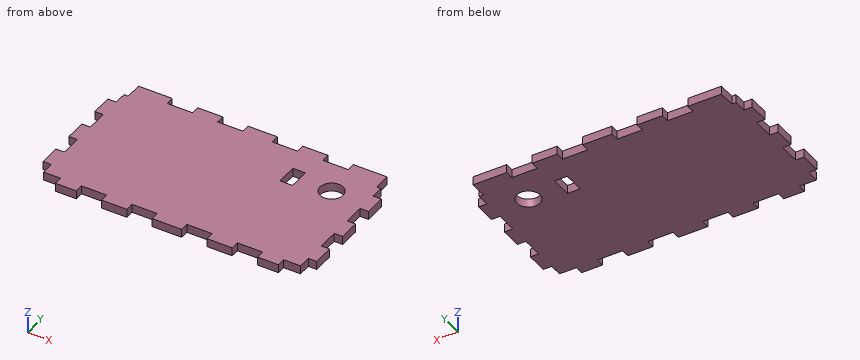
Autodesk Inventor part; units mm, degrees
ref_plane "YZ Plane" through (0, 0, 0) normal (1, 0, 0) x (0, 1, 0)
ref_plane "XZ Plane" through (0, 0, 0) normal (0, 1, 0) x (-1, 0, 0)
ref_plane "XY Plane" through (0, 0, 0) normal (0, 0, 1) x (1, 0, 0)
sketch "Sketch1" plane through (0, 0, 0) normal (0, 0, 1) x (1, 0, 0)
  line L0 (0, -74) -> (130, -74)
  line L1 (130, -74) -> (130, 0)
  line L2 (130, 0) -> (0, 0)
  line L3 (0, 0) -> (0, -74)
  dimension "d228" = 130
  dimension "d229" = 74
extrude "Extrusion1" add sketch "Sketch1" against normal blind 4
sketch "Sketch2" plane through (0, 0, 0) normal (0, 0, 1) x (1, 0, 0)
  line L0 (0, -74) -> (0, 0)
  line L1 (0, -37) -> (130, -37)
  line L2 (130, 0) -> (130, -74)
  line L3 (65, 0) -> (65, -74)
  line L4 (130, -74) -> (0, -74)
  line L5 (22, -74) -> (12, -74)
  line L6 (12, -74) -> (12, -70)
  line L7 (22, -70) -> (22, -74)
  line L8 (46, -70) -> (46, -74)
  line L9 (46, -74) -> (34, -74)
  line L10 (34, -74) -> (34, -70)
  line L11 (72, -70) -> (72, -74)
  line L12 (72, -74) -> (58, -74)
  line L13 (58, -74) -> (58, -70)
  line L14 (0, -74) -> (130, -74)
  line L15 (96, -74) -> (84, -74)
  line L16 (84, -74) -> (84, -70)
  line L17 (96, -70) -> (96, -74)
  line L18 (118, -70) -> (118, -74)
  line L19 (118, -74) -> (108, -74)
  line L20 (108, -74) -> (108, -70)
  line L21 (0, -54) -> (4, -54)
  line L22 (4, -54) -> (4, -44)
  line L23 (4, -44) -> (0, -44)
  line L24 (0, -44) -> (0, -54)
  line L25 (0, -34) -> (4, -34)
  line L26 (4, -34) -> (4, -24)
  line L27 (4, -24) -> (0, -24)
  line L28 (0, -24) -> (0, -34)
  line L29 (0, 0) -> (0, -74)
  line L30 (130, -74) -> (130, 0)
  line L31 (130, 0) -> (130, -74)
  line L32 (0, -70) -> (12, -70)
  line L33 (22, -70) -> (34, -70)
  line L34 (46, -70) -> (58, -70)
  line L35 (72, -70) -> (84, -70)
  line L36 (96, -70) -> (108, -70)
  line L37 (118, -70) -> (130, -70)
  line L38 (0, 0) -> (0, -74)
  line L39 (6, 0) -> (6, -8)
  line L40 (22, -4) -> (22, 0)
  line L41 (46, -4) -> (46, 0)
  line L42 (46, 0) -> (34, 0)
  line L43 (34, 0) -> (34, -4)
  line L44 (72, -4) -> (72, 0)
  line L45 (72, 0) -> (58, 0)
  line L46 (58, 0) -> (58, -4)
  line L47 (96, -4) -> (96, 0)
  line L48 (108, 0) -> (108, -4)
  line L49 (96, 0) -> (84, 0)
  line L50 (84, 0) -> (84, -4)
  line L51 (0, -74) -> (0, 0)
  line L52 (130, 0) -> (130, -74)
  line L53 (130, -74) -> (130, 0)
  line L54 (22, -4) -> (34, -4)
  line L55 (46, -4) -> (58, -4)
  line L56 (72, -4) -> (84, -4)
  line L57 (96, -4) -> (108, -4)
  line L58 (130, -74) -> (130, 0)
  line L59 (130, 0) -> (130, -74)
  line L60 (130, 0) -> (130, -74)
  line L61 (130, -74) -> (130, 0)
  line L62 (0, -70) -> (4, -70)
  line L63 (4, -70) -> (4, -64)
  line L64 (4, -64) -> (0, -64)
  line L65 (0, -64) -> (0, -70)
  line L66 (0, -4) -> (4, -4)
  line L67 (4, -4) -> (4, -14)
  line L68 (4, -14) -> (0, -14)
  line L69 (0, -14) -> (0, -4)
  line L70 (130, -74) -> (130, 0)
  line L71 (130, -54) -> (126, -54)
  line L72 (126, -54) -> (126, -44)
  line L73 (126, -44) -> (130, -44)
  line L74 (130, -44) -> (130, -54)
  line L75 (126, -34) -> (126, -24)
  line L76 (130, -34) -> (126, -34)
  line L77 (126, -24) -> (130, -24)
  line L78 (130, -24) -> (130, -34)
  line L79 (130, 0) -> (130, -74)
  line L80 (130, 0) -> (130, -74)
  line L81 (130, -74) -> (130, 0)
  line L82 (130, -70) -> (126, -70)
  line L83 (126, -70) -> (126, -64)
  line L84 (126, -64) -> (130, -64)
  line L85 (130, -64) -> (130, -70)
  line L86 (130, -4) -> (126, -4)
  line L87 (126, -4) -> (126, -14)
  line L88 (126, -14) -> (130, -14)
  line L89 (130, -14) -> (130, -4)
  line L90 (130, 0) -> (0, 0)
  line L91 (6, -8) -> (0, -8)
  line L92 (124, 0) -> (124, -8)
  line L93 (124, -8) -> (130, -8)
  point P0 (58, -74)
  point P1 (72, -74)
  point P2 (0, -24)
  point P3 (0, -34)
  point P4 (84, -74)
  point P5 (96, -74)
  point P6 (0, -44)
  point P7 (130, -70)
  point P8 (0, -70)
  point P9 (0, -14)
  point P10 (0, -64)
  point P11 (126, -70)
  point P12 (130, -64)
  point P13 (130, -54)
  point P14 (130, -44)
  point P15 (130, -34)
  point P16 (130, -14)
  point P17 (0, -8)
  point P18 (126, -8)
  dimension "d234" = 10
  dimension "d235" = 12
  dimension "d236" = 12
  dimension "d237" = 12
  dimension "d238" = 14
  dimension "d240" = 12
  dimension "d242" = 12
  dimension "d243" = 10
  dimension "d244" = 12
  dimension "d245" = 12
  dimension "d246" = 12
  dimension "d249" = 10
  dimension "d251" = 10
  dimension "d255" = 10
  dimension "d262" = 4
  dimension "d267" = 10
  dimension "d268" = 10
  dimension "d271" = 10
  dimension "d272" = 14
  dimension "d274" = 6
  dimension "d278" = 8
extrude "Extrusion2" cut sketch "Sketch2" against normal blind 4 contours L0 L32 L6 L4 | L0 L64 L63 L32 | L7 L33 L10 L4 | L0 L23 L22 L21 | L8 L34 L13 L4 | L0 L27 L26 L25 | L11 L35 L16 L4 | L0 L91 L67 L68 | L76 L75 L77 L2 | L2 L71 L72 L73 | L90 L50 L56 L44 | L46 L55 L41 L90 | L0 L66 L67 L91 | L17 L36 L20 L4 | L0 L90 L39 L91 L67 L66 | L88 L87 L93 L2 | L2 L37 L83 L84 | L90 L48 L57 L47 | L43 L54 L40 L90 | L93 L87 L86 L2 | L2 L4 L18 L37 | L86 L87 L93 L92 L90 L2
sketch "Sketch3" plane through (0, 0, -4) normal (0, 0, -1) x (-1, 0, 0)
  circle A0 centre (-110, -20) radius 5.5
  line L0 (-130, -14) -> (-130, -24)
  line L1 (-108, 0) -> (-124, 0)
  point P0 (0, 0)
  dimension "d279" = 11
  dimension "d280" = 20
  dimension "d281" = 20
extrude "Extrusion3" cut sketch "Sketch3" against normal blind 4
sketch "Sketch4" plane through (0, 0, -4) normal (0, 0, -1) x (-1, 0, 0)
  line L0 (-94.5, -15) -> (-88.5, -15)
  line L1 (-88.5, -15) -> (-88.5, -25)
  line L2 (-88.5, -25) -> (-94.5, -25)
  line L3 (-94.5, -25) -> (-94.5, -15)
  circle A0 centre (-110, -20) radius 5.5
  point P0 (0, 0)
  point P1 (-94.5, -20)
  dimension "d297" = 10
  dimension "d298" = 10
  dimension "d299" = 6
extrude "Extrusion4" cut sketch "Sketch4" against normal blind 4 contours L0 L1 L2 L3
properties part number "Langbektang houder"
CAD build for the part. Positions are in the model's coordinates, mm. Coordinates: 2 decimals unless noted, no trailing zeros. Order: outer loops, then holes, each group sorted by start corner. A loop starts at its lowest first (then second) coordinate and runs counter-clockwise, first axis right, second up. Notation, with made-up numbers: (-24, 22) -> (33, 22) arc R21 ccw to (33, 39) -> close; hole circle Ø9 at (50.25, 65.5). An arc over 180 degrees is marked (long way). Use one line per item in the form item = value. Start each with the question number.
1) Drill centre lines: L1, parallel to Y at x = 110, z = -1.85; L2, parallel to X at y = -19.5, z = -0.3; L3, parallel to X at y = -16, z = -0.5. Where is each one in solid material? Low to high. Write a range as [from, to].
2) Band-saw the part on C-C on z = -3.35. State how many separate pieces and enclosed holes the cut face has, then the cut area to 3 significant figures.
3) Band-saw the part on A-A on y = -20. Give the cut face in (x, z), then the cut area to 3 significant figures.
4) Drop flat-ended pins along their axis: pin 1 (2 mm diameter, centred on y = -4.5, z = -2.5, fed in from +X); pin 2 (2 mm diameter, centred on y = -46.5, z = -1, fed in from +X); pin 3 (2 mm diameter, centred on x = 79, z = -2, fed in from -Y). Give the stop position or say it passes through.
5) Band-saw the part on D-D on x = 32. Give the cut face in (y, z), then the cut area to 3 significant figures.
6) Band-saw the part on B-B on x = 110. Give the cut face in (y, z).
Entries:
q1.L1 = [-74, -25.5], [-14.5, 0]
q1.L2 = [0, 88.5], [94.5, 104.52], [115.48, 130]
q1.L3 = [0, 88.5], [94.5, 106.23], [113.77, 130]
q2.separate_pieces = 1
q2.enclosed_holes = 2
q2.area = 8,630 mm2
q3.outline = (0, -4) -> (88.5, -4) -> (88.5, 0) -> (0, 0) -> close; (94.5, -4) -> (104.5, -4) -> (104.5, 0) -> (94.5, 0) -> close; (115.5, -4) -> (130, -4) -> (130, 0) -> (115.5, 0) -> close
q3.area = 452 mm2
q4.pin_1 = 124
q4.pin_2 = 126
q4.pin_3 = -70
q5.outline = (-70, -4) -> (-4, -4) -> (-4, 0) -> (-70, 0) -> close
q5.area = 264 mm2
q6.outline = (-74, -4) -> (-25.5, -4) -> (-25.5, 0) -> (-74, 0) -> close; (-14.5, -4) -> (0, -4) -> (0, 0) -> (-14.5, 0) -> close
